Check sheet for the modelled part. Datum: model origin and axes. Units: mm. A direction names the side the tool comes from. Coordinates: 2 decimals unless noted, no trailing zeros. Order: outer loops, then holes, each group sorted by start corner. A loop starts at its lowest first (then second) coordinate and runs counter-clockwise, first axis right, second up. Notation, with made-up numbers: (12, 57) -> (45, 57) arc R29 ccw to (45, 86) -> close; hole circle Ø1 at (56.25, 43). An arc over 180 degrees is marked (long way). Put each result on its own line as item: value. Start each with the question number.
```python
from build123d import *

# Parameters (mm, degrees)
F1_DEPTH = 609.6


with BuildPart() as f1:
    # F0 (on Top) → F1 (new body)
    with BuildSketch(Plane.XY):
        with BuildLine():
            Line((0, 1219.2), (0, 0))
            Line((0, 0), (25.4, 0))
            Line((25.4, 0), (25.4, 12.7))
            Line((25.4, 12.7), (25.4, 139.7))
            Line((25.4, 139.7), (25.4, 190.5))
            Line((25.4, 190.5), (25.4, 317.5))
            Line((25.4, 317.5), (25.4, 368.3))
            Line((25.4, 368.3), (25.4, 495.3))
            Line((25.4, 495.3), (25.4, 546.1))
            ThreePointArc((25.4, 546.1), (32.839488, 564.060512), (50.8, 571.5))
            ThreePointArc((50.8, 571.5), (88.9, 609.6), (50.8, 647.7))
            ThreePointArc((50.8, 647.7), (32.839488, 655.139488), (25.4, 673.1))
            Line((25.4, 673.1), (25.4, 723.9))
            Line((25.4, 723.9), (25.4, 850.9))
            Line((25.4, 850.9), (25.4, 901.7))
            Line((25.4, 901.7), (25.4, 1028.7))
            Line((25.4, 1028.7), (25.4, 1079.5))
            Line((25.4, 1079.5), (25.4, 1206.5))
            Line((25.4, 1206.5), (25.4, 1219.2))
            Line((25.4, 1219.2), (0, 1219.2))
        make_face()
        with BuildLine():
            Line((25.4, 139.7), (25.4, 12.7))
            ThreePointArc((25.4, 12.7), (32.839488, 30.660512), (50.8, 38.1))
            ThreePointArc((50.8, 38.1), (88.9, 76.2), (50.8, 114.3))
            ThreePointArc((50.8, 114.3), (32.839488, 121.739488), (25.4, 139.7))
        make_face()
        with BuildLine():
            ThreePointArc((50.8, 1181.1), (32.839488, 1188.539488), (25.4, 1206.5))
            Line((25.4, 1206.5), (25.4, 1079.5))
            ThreePointArc((25.4, 1079.5), (32.839488, 1097.460512), (50.8, 1104.9))
            ThreePointArc((50.8, 1104.9), (88.9, 1143), (50.8, 1181.1))
        make_face()
        with BuildLine():
            Line((25.4, 317.5), (25.4, 190.5))
            ThreePointArc((25.4, 190.5), (32.839488, 208.460512), (50.8, 215.9))
            ThreePointArc((50.8, 215.9), (88.9, 254), (50.8, 292.1))
            ThreePointArc((50.8, 292.1), (32.839488, 299.539488), (25.4, 317.5))
        make_face()
        with BuildLine():
            ThreePointArc((50.8, 1003.3), (32.839488, 1010.739488), (25.4, 1028.7))
            Line((25.4, 1028.7), (25.4, 901.7))
            ThreePointArc((25.4, 901.7), (32.839488, 919.660512), (50.8, 927.1))
            ThreePointArc((50.8, 927.1), (88.9, 965.2), (50.8, 1003.3))
        make_face()
        with BuildLine():
            Line((25.4, 495.3), (25.4, 368.3))
            ThreePointArc((25.4, 368.3), (32.839488, 386.260512), (50.8, 393.7))
            ThreePointArc((50.8, 393.7), (88.9, 431.8), (50.8, 469.9))
            ThreePointArc((50.8, 469.9), (32.839488, 477.339488), (25.4, 495.3))
        make_face()
        with BuildLine():
            ThreePointArc((50.8, 825.5), (32.839488, 832.939488), (25.4, 850.9))
            Line((25.4, 850.9), (25.4, 723.9))
            ThreePointArc((25.4, 723.9), (32.839488, 741.860512), (50.8, 749.3))
            ThreePointArc((50.8, 749.3), (88.9, 787.4), (50.8, 825.5))
        make_face()
    extrude(amount=F1_DEPTH)


solid = f1.part
```
1) Scan lines: line 1 along X through (y, z) = (180, 177); line 2 along X through (y, z) = (592, 204.5). Record each from-to range of solid material in increasing order. Write a range as [from, to].
2) Access from +Z, -Z, +X, -X, +Y, -Y to the whole of each face (thin tool, end or side, straight path). Record for faces 1 (the cylindrical face through (33.04, 654.94, 300.53)), 2 (the flat face through (13, 0, 301)).
3) Gauge pin test, flat ends, axial feed: pin 1 (10 mm diameter, centred on y = 426, z = 321, fed in from +X); pin 2 (1 mm diameter, centred on x = 35, z = 533, fed in from +Y); pin 3 (1.5 mm diameter, centred on y = 193, z = 440.5, fed in from -X); pin 4 (8 mm diameter, centred on y = 1093.5, z = 359.5, fed in from +X). Record the tip position at first contact, or that the pin passes through.
4) Mould release check, pull along Y, two halves, no side actions. Record for faces 3 (the cylindrical face through (33.04, 1010.54, 300.53)), 4 (the flat face through (34, 618, 0)), 5 (the cylindrical face through (33.04, 1188.34, 300.53)), 6 (the cylindrical face through (88.89, 964.36, 300.53)): +Y half, -Y half, draft (parallel to the pull), parting line (faces both ways), or undercut.
5) Sectioned sample at B-B (y = 883). Record the boundary of the cut face in (x, z), plus the area to 3 significant figures.
6) Sectioned sample at C-C (y = 1116). Record the boundary of the cut face in (x, z), plus the area to 3 significant figures.
Entries:
1. line 1: x = [0, 25.4]
1. line 2: x = [0, 84.59]
2. face 1: +Z, -Z, +X
2. face 2: +Z, -Z, +X, -X, -Y
3. pin 1: stops at x = 88.89
3. pin 2: stops at y = 1187.02
3. pin 3: stops at x = 0
3. pin 4: stops at x = 32.88
4. face 3: undercut
4. face 4: draft
4. face 5: +Y half
4. face 6: undercut
5. outline: (0, 0) -> (25.4, 0) -> (25.4, 609.6) -> (0, 609.6) -> close
5. area: 15,500 mm2
6. outline: (0, 0) -> (77.68, 0) -> (77.68, 609.6) -> (0, 609.6) -> close
6. area: 47,400 mm2
